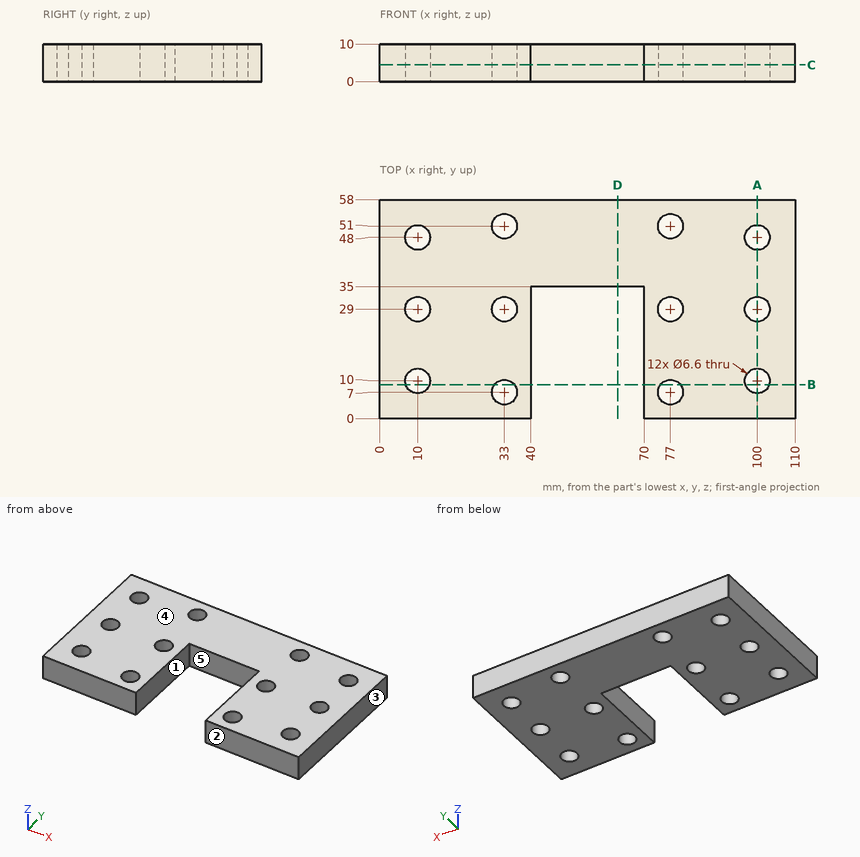
The figure shows three views and two pictorial views of one solid part (mm, origin at its lowest corner). Answer the questions. A direction names the side the tool comes from. Round coordinates to 2 decimals unless told otherwise and drop trailing zeros. Write each loop counter-clockwise with the first axis right and the second up, starting at its lowest first coordinate (ties: lowest second). Pieces come first, ordered by that corner, then holes. Notation, with made-up numbers: (12, 5) - (17, 5) arc R4 cw to (17, 12) - close; hole circle Ø6 at (-30, 59.25). An arc over 180 degrees is marked (long way). Answer in a Markdown table with one row per item. Add a question column.
1. A cutting plane is placed at A-A, the plane x = 100. Determine the outline of the cut face in (y, z), and give its area (3 significant figures).
2. A cutting plane is placed at C-C, the plane z = 4.5. Count the separate pieces of the cut face and the enclosed holes in it, and give its area (3 significant figures).
3. Given pin 1 (5 mm diameter, centred on x = 50.5, z = 6, fed in from -Y), flat-ended and moving along its own axis, determine where the tip first touches the part or whether it passes through.
4. A cutting plane is placed at B-B, the plane y = 9. Determine the outline of the cut face in (x, z).
5. Find the intervals of material crossed by line 1 along Y through (x, z) = (77, 6.75); line 2 along X through (y, z) = (29, 4.5); line 3 along X through (y, z) = (14.5, 7.25), in increasing order. Write a range as from..to.
6. A cutting plane is placed at D-D, the plane x = 63. Determine the outline of the cut face in (y, z).
7. The mould has two halves that part along X. Classify the marked faces 1, 2 and 3: +X half, -X half, draft (parallel to the pull), parting line (faces both ways), or undercut.
8. For the marked faces 4 and 5, determine the directions among +Z, -Z, +X, -X, +Y, -Y from which every point of the face is accessible in a straight line to the end or side of a thin tool.
Worked out:
| question | item | result |
|---|---|---|
| 1 | outline | (0, 0) - (6.7, 0) - (6.7, 10) - (0, 10) - close; (13.3, 0) - (25.7, 0) - (25.7, 10) - (13.3, 10) - close; (32.3, 0) - (44.7, 0) - (44.7, 10) - (32.3, 10) - close; (51.3, 0) - (58, 0) - (58, 10) - (51.3, 10) - close |
| 1 | area | 382 mm^2 |
| 2 | separate pieces | 1 |
| 2 | enclosed holes | 12 |
| 2 | area | 4,920 mm^2 |
| 3 | pin 1 | y = 35 |
| 4 | outline | (0, 0) - (6.86, 0) - (6.86, 10) - (0, 10) - close; (13.14, 0) - (30.38, 0) - (30.38, 10) - (13.14, 10) - close; (35.62, 0) - (40, 0) - (40, 10) - (35.62, 10) - close; (70, 0) - (74.38, 0) - (74.38, 10) - (70, 10) - close; (79.62, 0) - (96.86, 0) - (96.86, 10) - (79.62, 10) - close; (103.14, 0) - (110, 0) - (110, 10) - (103.14, 10) - close |
| 5 | line 1 | 0..3.7, 10.3..25.7, 32.3..47.7, 54.3..58 |
| 5 | line 2 | 0..6.7, 13.3..29.7, 36.3..40, 70..73.7, 80.3..96.7, 103.3..110 |
| 5 | line 3 | 0..40, 70..110 |
| 6 | outline | (35, 0) - (58, 0) - (58, 10) - (35, 10) - close |
| 7 | face 1 | undercut |
| 7 | face 2 | draft |
| 7 | face 3 | +X half |
| 8 | face 4 | +Z, +X, -X, +Y, -Y |
| 8 | face 5 | +Z, -Z, -Y |
